Geometry check sheet. Reference: the model listing, model coordinates, mm. A direction names the side the tool comes from. Give positions to 0.01 mm unless a question says otherwise; leave off trailing zeros. Order: outer loops, then holes, each group sorted by start corner. A loop starts at its lowest first (then second) coordinate and runs counter-clockwise, first axis right, second up. Notation, with made-up numbers: M -28,52 L 31,52 A21 ccw 31,83 Z; hole C 67.25,21.25 d4. An arc over 180 degrees is marked long. Answer as a JSON object with one key per item and string values. Group by question number.
from build123d import *

# Parameters (mm, degrees)
F0_W     = 1000
F0_H     = 1000
F1_DEPTH = 500
F3_T     = -10
F2_W     = 300
F2_H     = 300
F4_DEPTH = 100
F5_T     = -10


# Not quite as in the source:
# - a shell that OpenCascade refuses in one call is made with other operations: the cavity is built on its own and cut out


with BuildPart() as f1:
    # F0 (on Top) → F1 (new body)
    with BuildSketch(Plane.XY):
        Rectangle(F0_W, F0_H)
    extrude(amount=F1_DEPTH)

    # F3
    f3_openings = [f1.faces().sort_by_distance(p)[0] for p in [
        (0, 0, 0),
    ]]
    offset(amount=F3_T, openings=f3_openings)

    # F2 (on face) → F4 (join)
    with BuildSketch(Plane.XY.offset(500)):
        Rectangle(F2_W, F2_H)
    extrude(amount=F4_DEPTH)

    # F5: a shell. OpenCascade refuses it in one call, so the cavity is built on its own and cut out:
    # the body offset inwards by the wall thickness, plus a prism from it out through each open face.
    f5_core = offset(f1.part, amount=F5_T, kind=Kind.INTERSECTION, mode=Mode.PRIVATE)
    f5_exits = [f5_core.faces().sort_by_distance(p)[0] for p in [
        (0, 0, 590),
    ]]
    add(f5_core, mode=Mode.SUBTRACT)
    extrude(f5_exits, amount=-F5_T, mode=Mode.SUBTRACT)


solid = f1.part
1. Thickness scan on line 1 along X through (y, z) = (82, 146); line 2 along Y through (x, z) = (15, 505). Record the ranges inside material, lowest first. Write a range as [from, to].
2. Cross-section at A-A (z = 123.5). Record the cut outline in (x, y).
3. Depth check by flat-ended pin: pin 1 (12 mm diameter, centred on x = 156.5, y = 319, fed in from +Z). Enter the tip coordinate at first touch or a pass-through.
4. Cross-section at B-B (x = -85). Record the cut outline in (y, z), and give its area (3 significant figures).
5. Cross-section at C-C (y = 313). Record the cut outline in (x, z).
6. Access from +Z, -Z, +X, -X, +Y, -Y to the whole of each face (thin tool, end or side, straight path). Record for faces 1 (the flat face through (-2, -150, 549)), 2 (the flat face through (-2, -140, 549)), 3 (the flat face through (-490, -7, 242)), 4 (the flat face through (-2, 150, 549)).
7. Cross-section at D-D (z = 519.5). Record the cut outline in (x, y), and give its area (3 significant figures).
8. Release check for a two-part mould opening along X. For faces 5 (the flat face through (150, -2, 549)), 6 (the flat face through (-7, 490, 242)), 7 (the flat face through (-500, -7, 246)) record: released by +X, released by -X, zero draft, split by the parting line, or undercut.
Report:
{
 "1": {"line 1": "x = [-500, -490], [490, 500]", "line 2": "y = [-150, -140], [140, 150]"},
 "2": {"outline": "M -500,-500 L 500,-500 L 500,500 L -500,500 Z; hole M -490,-490 L 490,-490 L 490,490 L -490,490 Z"},
 "3": {"pin 1": "stops at z = 500"},
 "4": {"outline": "M -500,0 L -490,0 L -490,490 L 490,490 L 490,0 L 500,0 L 500,500 L 150,500 L 150,600 L 140,600 L 140,500 L -140,500 L -140,600 L -150,600 L -150,500 L -500,500 Z", "area": "21,800 mm2"},
 "5": {"outline": "M -500,0 L -490,0 L -490,490 L 490,490 L 490,0 L 500,0 L 500,500 L -500,500 Z"},
 "6": {"face 1": "+Z, +X, -X, -Y", "face 2": "+Z", "face 3": "-Z", "face 4": "+Z, +X, -X, +Y"},
 "7": {"outline": "M -150,-150 L 150,-150 L 150,150 L -150,150 Z; hole M -140,-140 L 140,-140 L 140,140 L -140,140 Z", "area": "11,600 mm2"},
 "8": {"face 5": "released by +X", "face 6": "undercut", "face 7": "released by -X"}
}
